from build123d import *
from OCP.BRepFilletAPI import BRepFilletAPI_MakeChamfer

# Parameters (mm, degrees)
SKETCH1_W           = 60
SKETCH1_H           = 50
BOSS_EXTRUDE1_DEPTH = 15
CHAMFER1_SIZE       = 10
CHAMFER1_SIZE2      = 5.773502692
SKETCH2_W           = 20
SKETCH2_H           = 30
CUT_EXTRUDE1_DEPTH  = 5


with BuildPart() as part:
    # Sketch1 → Boss-Extrude1 (new body)
    with BuildSketch(Plane(origin=(0, 0, 0), x_dir=(1, 0, 0), z_dir=(0, 1, 0))):
        Rectangle(SKETCH1_W, SKETCH1_H)
    extrude(amount=BOSS_EXTRUDE1_DEPTH)

    # Chamfer1: one chamfer whose edges measure the first distance from different faces: ONE call of the kernel's chamfer builder (chamfer() names one face for all edges)
    chamfer1_edges_1 = [part.edges().sort_by_distance(p)[0] for p in [
        (30, 7.5, 25),
    ]]
    chamfer1_side_1 = [part.faces().sort_by_distance(p)[0] for p in [
        (0, 7.5, 25),
    ]]
    chamfer1_edges_2 = [part.edges().sort_by_distance(p)[0] for p in [
        (-30, 7.5, 25),
    ]]
    chamfer1_side_2 = [part.faces().sort_by_distance(p)[0] for p in [
        (-30, 7.5, 0),
    ]]
    chamfer1_edges_3 = [part.edges().sort_by_distance(p)[0] for p in [
        (-30, 7.5, -25),
    ]]
    chamfer1_side_3 = [part.faces().sort_by_distance(p)[0] for p in [
        (0, 7.5, -25),
    ]]
    chamfer1_edges_4 = [part.edges().sort_by_distance(p)[0] for p in [
        (30, 7.5, -25),
    ]]
    chamfer1_side_4 = [part.faces().sort_by_distance(p)[0] for p in [
        (30, 7.5, 0),
    ]]
    chamfer1 = BRepFilletAPI_MakeChamfer(part.part.solid().wrapped)
    for e in chamfer1_edges_1:
        chamfer1.Add(CHAMFER1_SIZE, CHAMFER1_SIZE2, e.wrapped, chamfer1_side_1[0].wrapped)  # the first distance lies on this face
    for e in chamfer1_edges_2:
        chamfer1.Add(CHAMFER1_SIZE, CHAMFER1_SIZE2, e.wrapped, chamfer1_side_2[0].wrapped)  # the first distance lies on this face
    for e in chamfer1_edges_3:
        chamfer1.Add(CHAMFER1_SIZE, CHAMFER1_SIZE2, e.wrapped, chamfer1_side_3[0].wrapped)  # the first distance lies on this face
    for e in chamfer1_edges_4:
        chamfer1.Add(CHAMFER1_SIZE, CHAMFER1_SIZE2, e.wrapped, chamfer1_side_4[0].wrapped)  # the first distance lies on this face
    add(Compound.cast(chamfer1.Shape()), mode=Mode.REPLACE)

    # Sketch2 → Cut-Extrude1 (cut)
    with BuildSketch(Plane(origin=(0, 15, 0), x_dir=(1, 0, 0), z_dir=(0, 1, 0))):
        Polygon((30, 15), (24.226497308, 25), (-20, 25), (-30, 19.226497308), (-30, -15), (-24.226497308, -25), (20, -25), (30, -19.226497308), align=None)
        Rectangle(SKETCH2_W, SKETCH2_H, mode=Mode.SUBTRACT)
    extrude(amount=-CUT_EXTRUDE1_DEPTH, mode=Mode.SUBTRACT)


solid = part.part
Verification items for the finished model (mm, model axes). A direction names the side the tool comes from. Coordinates: 2 decimals unless noted, no trailing zeros. Write each loop counter-clockwise with the first axis right and the second up, starting at its lowest first coordinate (ties: lowest second). Pieces come first, ordered by that corner, then holes. Notation, with made-up numbers: M 55.25,54 L 102.25,54 A23 cw 102.25,69 Z; hole C -3,67 d3. An arc over 180 degrees is marked long. Use CSV: the item, a comma, the result in double quotes.
Q1. Section check C-C, the plane z = -21. Enter the section's corners in (x, y).
Computed values:
outline,"M -26.93,0 L 26.54,0 L 26.54,10 L -26.93,10 Z"
Q2. Set-up check for faces 1 (the flat face through (0, 15, 0)), 2 (the flat face through (0, 13, -15)), 3 (the flat face through (0, 13, 15)), 4 (the flat face through (-10, 13, 0)), 5 (the flat face through (10, 13, 0)): record each of +Z, -Z, +X, -X, +Y, -Y from which the full face is reachable in a straight line by a thin tool's end or side.
Computed values:
face 1,"+Z, -Z, +X, -X, +Y"
face 2,"-Z, +X, -X, +Y"
face 3,"+Z, +X, -X, +Y"
face 4,"+Z, -Z, -X, +Y"
face 5,"+Z, -Z, +X, +Y"
Q3. Go/stop test with flat-tipped pins: P1, Ø5.5, axis at y = 13.5, z = -3, coming from the -X side; P2, Ø2.5, axis at y = 13.5, z = -5, coming from the +X side; P3, Ø1.5, axis at x = 3, y = 12, coming from the -Z side. Record where each tip stops, or that it passes through.
Computed values:
P1,"x = -10"
P2,"x = 10"
P3,"z = -15"
Q4. Section check D-D, the plane x = -14.5. Enter the section's corners in (y, z).
Computed values:
outline,"M 0,-25 L 10,-25 L 10,25 L 0,25 Z"
Q5. Section check A-A, the plane y = 8.25. Enter the section's corners in (x, z).
Computed values:
outline,"M -30,-19.23 L -20,-25 L 24.23,-25 L 30,-15 L 30,19.23 L 20,25 L -24.23,25 L -30,15 Z"
Q6. Thickness scan on line 1 along Y through (x, z) = (-27, 13); line 2 along X through (y, z) = (13, -11); line 3 along Z through (x, y) = (-3, 13). Record the ranges inside material, lowest first. Write a range as [from, to].
Computed values:
line 1,"[0, 10]"
line 2,"[-10, 10]"
line 3,"[-15, 15]"
Q7. Section check B-B, the plane x = 8. Enter the section's corners in (y, z), and give its area (3 significant figures).
Computed values:
outline,"M 0,-25 L 10,-25 L 10,-15 L 15,-15 L 15,15 L 10,15 L 10,25 L 0,25 Z"
area,"650 mm²"
